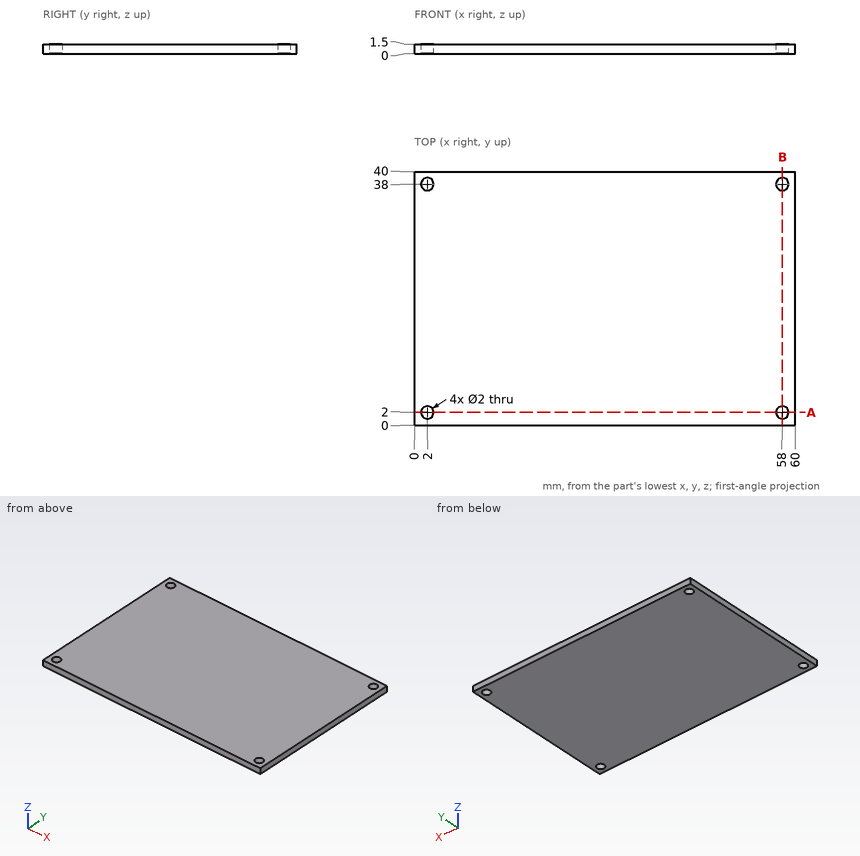
Geometry: see drawing. Coordinates: mm, zero at the bounding-box minimum. Coordinates: 2 decimals unless noted, no trailing zeros. Loops run counter-clockwise (first coordinate to the right, second up) from the corner with the lowest first, then second, coordinate; pieces in that order, holes last. Notation, with made-up numbers: (55.5, 34.25) - (62.5, 34.25) arc R20 ccw to (62.5, 52.25) - close; hole circle Ø8 at (31.5, -34). An arc over 180 degrees is marked (long way). Put each result on its own line as item: value. Start each with the question number.
Q1. Cut plane A-A, the plane y = 2. Return loops of the section in (x, z), and give its area (3 significant figures).
Q2. Line query: line 1 (X direction, y = 38, z = 1.05); line 2 (Y direction, x = 2, z = 0.8). Output: solid intervals per line, ascending.
Q3. Pin query (flat end, axial travel): pin 1 Ø1.6 at (x, y) = (2, 38) entering from +Z; pin 2 Ø3 at (x, y) = (2, 2) entering from +Z. Return the tip coordinate at first contact, or that it passes through.
Q4. Cut plane B-B, the plane x = 58. Return loops of the section in (y, z).
Filled sheet:
1. outline: (0, 0) - (1, 0) - (1, 1.5) - (0, 1.5) - close; (3, 0) - (57, 0) - (57, 1.5) - (3, 1.5) - close; (59, 0) - (60, 0) - (60, 1.5) - (59, 1.5) - close
1. area: 84.0 mm²
2. line 1: 0 to 1, 3 to 57, 59 to 60
2. line 2: 0 to 1, 3 to 37, 39 to 40
3. pin 1: through
3. pin 2: z = 1.5
4. outline: (0, 0) - (1, 0) - (1, 1.5) - (0, 1.5) - close; (3, 0) - (37, 0) - (37, 1.5) - (3, 1.5) - close; (39, 0) - (40, 0) - (40, 1.5) - (39, 1.5) - close
